Autodesk Inventor part; units mm, degrees
ref_plane "Work Plane1" through (0, 0, 0) normal (-1, 0, 0) x (0, 0, 1)
ref_plane "Work Plane5" through (0, 26.089513, 40) normal (-1, 0, 0) x (0, 0, 1)
ref_plane "Work Plane4" through (0, 60, 20) normal (-1, 0, 0) x (0, 0, 1)
sketch "Sketch1" plane through (0, 0, 0) normal (0, 1, 0) x (-1, 0, 0)
  line L0 (0, 0) -> (-30, 0)
  arc A0 (170, 89.262855) -> (-30, 108.626345) centre (58, -25) ccw
  line L1 (-30, 0) -> (-30, 108.626345)
  line L2 (0, 0) -> (0, 80.052368)
  arc A1 (150, 52.045441) -> (0, 80.052368) centre (58, -25) ccw
  line L3 (170, 30) -> (170, 89.262855)
  line L4 (170, 0) -> (150, 0)
  line L5 (150, 52.045441) -> (150, 30)
  line L6 (150, 30) -> (170, 30)
  point P0 (-8.450723, -25)
  point P1 (160, 30)
  point P2 (160, 0)
  dimension "d0" = 30
  dimension "d1" = 25
  dimension "d3" = 320
  dimension "d137" = 30
ref_plane "Work Plane1" through (0, 0, 0) normal (-1, 0, 0) x (0, 0, 1)
ref_plane "Work Plane5" through (0, 26.089513, 40) normal (-1, 0, 0) x (0, 0, 1)
ref_plane "Work Plane4" through (0, 60, 20) normal (-1, 0, 0) x (0, 0, 1)
ref_plane "Work Plane2" through (-170, 0, 89.262855) normal (-1, 0, 0) x (0, 0, 1)
sketch "Sketch7" plane through (-170, 0, 89.262855) normal (-1, 0, 0) x (0, 0, 1)
  point P0 (-89.262855, 0)
ref_plane "Work Plane3" through (-170, 0, 0) normal (-1, 0, 0) x (0, 0, 1)
extrude "Extrusion4" add sketch "Sketch1" along normal blind 25
sketch "Sketch9" plane through (0, 25, 0) normal (0, 1, 0) x (1, 0, 0)
  line L0 (-170, 0) -> (-170, -89.262855)
  line L1 (-170, -48) -> (-150, -48)
  line L2 (-150, 0) -> (-170, 0)
  line L3 (-150, -48) -> (-150, -52.484587)
  line L4 (-170, -48) -> (-170, -89.262855)
  arc A0 (-150, -52.045441) -> (0, -80.052368) centre (-58, 25) ccw
  arc A1 (-150, -52.045441) -> (0, -80.052368) centre (-58, 25) ccw
  arc A2 (-170, -89.262855) -> (30, -108.626345) centre (-58, 25) ccw
  arc A3 (-170, -89.262855) -> (30, -108.626345) centre (-58, 25) ccw
  line L5 (-0.01, 0) -> (-0.01, -80.052368)
  line L6 (-0.01, -80.057888) -> (-0.01, 0)
  line L7 (30, 0) -> (-0.01, 0)
  line L8 (-0.01, 0) -> (30, 0)
  line L9 (30, -108.626345) -> (30, 0)
  line L10 (30, 0) -> (30, -108.626345)
  point P0 (0, 0)
  dimension "d79" = 20
  dimension "d80" = 48
extrude "Extrusion5" add sketch "Sketch9" along normal blind 30
sketch "Sketch10" plane through (0, 55, 0) normal (0, 1, 0) x (1, 0, 0)
  arc A0 (-150, -52.045441) -> (0, -79.707213) centre (-58.395171, 24.165786) ccw
  arc A1 (-170, -89.262855) -> (30, -108.626345) centre (-58, 25) ccw
  arc A2 (-170, -89.262855) -> (30, -108.626345) centre (-58, 25) ccw
  arc A3 (-150, -52.045441) -> (0, -80.052368) centre (-58, 25) ccw
  line L0 (-0.01, 0) -> (-0.01, -80.052368)
  line L1 (0, -80.052368) -> (-0.01, 0)
  line L2 (30, 0) -> (-0.01, 0)
  line L3 (-0.01, 0) -> (30, 0)
  line L4 (30, -108.626345) -> (30, 0)
  line L5 (30, 0) -> (30, -108.626345)
  line L6 (-170, 0) -> (-150, 0)
  line L7 (-170, -30) -> (-170, -89.262855)
  line L8 (-170, -89.262855) -> (-170, -30)
  line L9 (-150, -30) -> (-170, -30)
  line L10 (-170, -30) -> (-150, -30)
  line L11 (-150, -30) -> (-150, -52.045441)
  line L12 (-150, -48) -> (-150, -30)
  point P0 (0, 0)
  point P1 (-59.337804, -94.992543)
  point P2 (-0.000043, -79.707237)
  point P3 (-0.01, -79.712834)
sketch "Sketch10 outline for Extrusion6" plane through (0, 55, 0) normal (0, 1, 0) x (1, 0, 0)
  arc A0 (-0.000043, -79.707237) -> (-59.337804, -94.992543) centre (-58.395171, 24.165786) cw
  line L0 (-0.01, 0) -> (-0.000043, -79.707237)
  line L1 (30, 0) -> (-0.01, 0)
  line L2 (30, -108.626345) -> (30, 0)
  arc A1 (-170, -89.262855) -> (30, -108.626345) centre (-58, 25) ccw
  line L3 (-170, -30) -> (-170, -89.262855)
  line L4 (-150, -30) -> (-170, -30)
  line L5 (-150, -52.045441) -> (-150, -30)
  arc A2 (-59.337804, -94.992543) -> (-150, -52.045441) centre (-58, 25) cw
extrude "Extrusion6" add sketch "Sketch10 outline for Extrusion6" along normal blind 25
sketch "Sketch11" plane through (-0.01, 25, 0) normal (-1, 0, 0) x (0, 0, 1)
  point P0 (0, -25)
sketch "Sketch14" plane through (-0.01, 25, 0) normal (-1, 0, 0) x (0, 0, 1)
  point P0 (0, -25)
chamfer "Chamfer7" distance 2 angle 45 1 edges at (14.995, 80, 0) measured on face at (20, 80, 62.7779)
chamfer "Chamfer8" distance 2 angle 45 1 edges at (15, 0, 0) measured on face at (20, 0, 62.8929)
sketch "Sketch16" plane through (30, 0, 108.626345) normal (1, 0, 0) x (0, 0, -1)
  circle A0 centre (68.626345, 60) radius 7.5
  circle A1 centre (88.626345, 60) radius 7.5
  circle A2 centre (88.626345, 20) radius 7.5
  circle A3 centre (68.626345, 20) radius 7.5
  line L0 (108.626345, 2) -> (108.626345, 78)
  line L1 (0, 80) -> (106.626345, 80)
  line L2 (0, 0) -> (106.626345, 0)
  point P0 (108.626345, 0)
  dimension "d138" = 15
  dimension "d139" = 15
  dimension "d140" = 15
  dimension "d141" = 15
  dimension "d142" = 20
  dimension "d143" = 20
  dimension "d144" = 20
  dimension "d145" = 20
  dimension "d146" = 20
  dimension "d147" = 20
  dimension "d148" = 20
  dimension "d149" = 20
hole "Hole7" at (30, 20, 40) at (30, 60, 40) at (30, 60, 20) at (30, 20, 20) direction (-1, 0, 0) diameter 15 depth 8
sketch "Sketch17" plane through (30, 0, 108.626345) normal (1, 0, 0) x (0, 0, -1)
  circle A0 centre (68.626345, 60) radius 4.2
  circle A1 centre (68.626345, 20) radius 4.2
  circle A2 centre (88.626345, 20) radius 7.5
  circle A3 centre (88.626345, 20) radius 4.2
  circle A4 centre (88.626345, 60) radius 7.5
  circle A5 centre (88.626345, 60) radius 4.2
  line L0 (108.626345, 2) -> (108.626345, 78)
  line L1 (0, 80) -> (106.626345, 80)
  line L2 (0, 0) -> (106.626345, 0)
  point P0 (108.626345, 0)
  dimension "d157" = 8.4
  dimension "d158" = 8.4
  dimension "d159" = 8.4
  dimension "d160" = 8.4
  dimension "d161" = 40
  dimension "d162" = 20
  dimension "d163" = 40
  dimension "d164" = 20
hole "Hole8" at (30, 60, 40) at (30, 20, 40) at (30, 20, 20) at (30, 60, 20) direction (-1, 0, 0) diameter 8.4 depth 50
sketch "Sketch18" plane through (-170, 0, 30) normal (-1, 0, 0) x (0, 0, 1)
  circle A0 centre (15, 17.5) radius 4
  circle A1 centre (15, 62.5) radius 4
  line L0 (0, 0) -> (0, 25)
  line L1 (0, 55) -> (0, 80)
  line L2 (0, 0) -> (59.262855, 0)
  line L3 (0, 80) -> (59.262855, 80)
  point P0 (-30, 0)
  dimension "d172" = 8
  dimension "d173" = 8
  dimension "d174" = 15
  dimension "d175" = 15
  dimension "d176" = 17.5
  dimension "d177" = 17.5
  dimension "d178" = 45
hole "Hole9" at (-170, 17.5, 45) at (-170, 62.5, 45) direction (1, 0, 0) diameter 8 depth 12 tip angle 118
properties part number "Gestell" material "Steel, Mild"
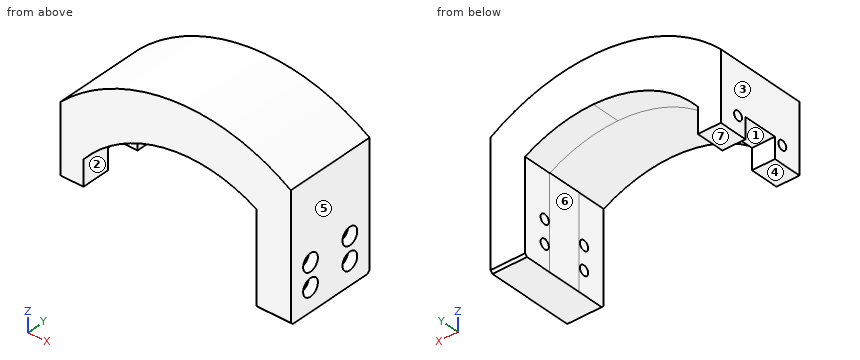
Geometry check sheet. Reference: the model listing, model coordinates, mm. Face numbers are marked on the shaded views. A direction names the side the tool comes from. Give positions to 0.01 mm unless a question says otherwise; leave off trailing zeros. Write each loop counter-clockwise with the first axis right and the second up, starting at its lowest first coordinate (ties: lowest second). Pieces come first, ordered by that corner, then holes. Notation, with made-up numbers: M 49.5,-16.5 L 90.5,-16.5 A23 ccw 90.5,22.5 Z; hole C 17,37.5 d4. An arc over 180 degrees is marked long. One line per question, with ' | ' between items.
1. Cross-section at B-B (y = 5). Enter the section's corners in (x, z), plus the area to 3 significant figures.
Ans:
outline: M -170,30 L -150,30 L -150,52.05 A120 cw 0,80.05 L 0,0 L 30,0 L 30,108.63 A160 ccw -170,89.26 Z | area: 11,300 mm2
2. Gauge pin test, flat ends, axial feed: pin 1 (10 mm diameter, centred on x = -157, y = 47, fed in from -Z); pin 2 (13.5 mm diameter, centred on y = 60, z = 40, fed in from +X); pin 3 (9 mm diameter, centred on y = 38, z = 43, fed in from -X); pin 4 (7.5 mm diameter, centred on y = 60, z = 20, fed in from +X). Record the tip position at first contact, or that the pin passes through.
Ans:
pin 1: z = 48 | pin 2: x = 22 | pin 3: x = -0.01 | pin 4: through
3. Scan lines: line 1 along Y through (x, z) = (16.5, 40); line 2 along Y through (x, z) = (24.5, 20); line 3 along Y through (x, z) = (-163.25, 45). Record each from-to range of solid material in increasing order. Write a range as from..to.
Ans:
line 1: 0..15.8, 24.2..55.8, 64.2..80 | line 2: 0..12.5, 27.5..52.5, 67.5..80 | line 3: 0..13.5, 21.5..25, 55..58.5, 66.5..80
4. Cross-section at C-C (x = -83.5). Enter the section's corners in (y, z), plus the area to 3 significant figures.
Ans:
outline: M 0,92.26 L 80,92.26 L 80,132.95 L 0,132.95 Z | area: 3,260 mm2
5. Set-up check for the marked faces 1, 2, 3 and 4: record each of +Z, -Z, +X, -X, +Y, -Y from which the full face is reachable in a straight line by a thin tool's end or side.
Ans:
face 1: -Z, -X | face 2: -Z, +Y, -Y | face 3: +Z, -Z, -X, +Y, -Y | face 4: -Z, -X, +Y, -Y
6. Mould release check, pull along X, two halves, no side actions. Record for the marked faces 5, 6 and 7: released by +X, released by -X, zero draft, split by the parting line, or undercut.
Ans:
face 5: released by +X | face 6: undercut | face 7: zero draft
